Geometry: final body of the model. Coordinates: model frame, mm. Give positions to 0.01 mm unless a question says otherwise; leave off trailing zeros. One line per question, with ' | ' between items.
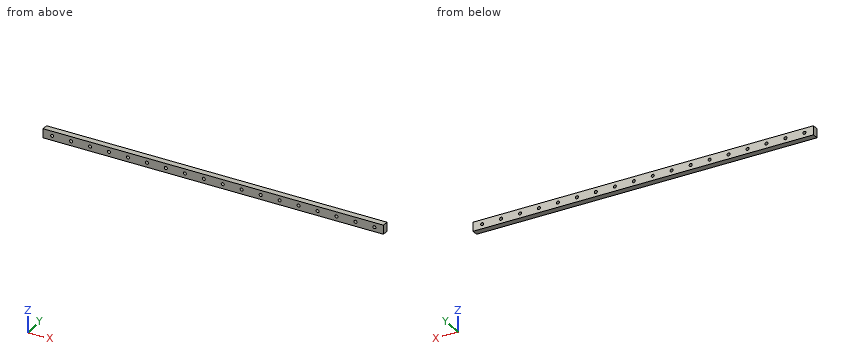
from build123d import *

# Parameters (mm, degrees)
SKETCH1_W           = 449
SKETCH1_H           = 12
SKETCH1_R           = 2
BOSS_EXTRUDE1_DEPTH = 8


with BuildPart() as part:
    # Sketch1 → Boss-Extrude1 (new body)
    with BuildSketch(Plane(origin=(0, 0, 0), x_dir=(1, 0, 0), z_dir=(0, 1, 0))):
        with Locations((224.5, 6)):
            Rectangle(SKETCH1_W, SKETCH1_H)
        with Locations(Location((12, 6, 0), (0, 0, 270))):
            Circle(SKETCH1_R, mode=Mode.SUBTRACT)
        with Locations(Location((37, 6, 0), (0, 0, 270))):
            Circle(SKETCH1_R, mode=Mode.SUBTRACT)
        with Locations(Location((62, 6, 0), (0, 0, 270))):
            Circle(SKETCH1_R, mode=Mode.SUBTRACT)
        with Locations(Location((87, 6, 0), (0, 0, 270))):
            Circle(SKETCH1_R, mode=Mode.SUBTRACT)
        with Locations(Location((112, 6, 0), (0, 0, 270))):
            Circle(SKETCH1_R, mode=Mode.SUBTRACT)
        with Locations(Location((137, 6, 0), (0, 0, 270))):
            Circle(SKETCH1_R, mode=Mode.SUBTRACT)
        with Locations(Location((162, 6, 0), (0, 0, 270))):
            Circle(SKETCH1_R, mode=Mode.SUBTRACT)
        with Locations(Location((187, 6, 0), (0, 0, 270))):
            Circle(SKETCH1_R, mode=Mode.SUBTRACT)
        with Locations(Location((212, 6, 0), (0, 0, 270))):
            Circle(SKETCH1_R, mode=Mode.SUBTRACT)
        with Locations(Location((237, 6, 0), (0, 0, 270))):
            Circle(SKETCH1_R, mode=Mode.SUBTRACT)
        with Locations(Location((262, 6, 0), (0, 0, 270))):
            Circle(SKETCH1_R, mode=Mode.SUBTRACT)
        with Locations(Location((287, 6, 0), (0, 0, 270))):
            Circle(SKETCH1_R, mode=Mode.SUBTRACT)
        with Locations(Location((312, 6, 0), (0, 0, 270))):
            Circle(SKETCH1_R, mode=Mode.SUBTRACT)
        with Locations(Location((337, 6, 0), (0, 0, 270))):
            Circle(SKETCH1_R, mode=Mode.SUBTRACT)
        with Locations(Location((362, 6, 0), (0, 0, 270))):
            Circle(SKETCH1_R, mode=Mode.SUBTRACT)
        with Locations(Location((387, 6, 0), (0, 0, 270))):
            Circle(SKETCH1_R, mode=Mode.SUBTRACT)
        with Locations(Location((412, 6, 0), (0, 0, 270))):
            Circle(SKETCH1_R, mode=Mode.SUBTRACT)
        with Locations(Location((437, 6, 0), (0, 0, 270))):
            Circle(SKETCH1_R, mode=Mode.SUBTRACT)
    extrude(amount=BOSS_EXTRUDE1_DEPTH)


solid = part.part
1) Material intervals for probe 1 along Z at (x, y) = (162, 5.75), sorted ascending. Write a range as from..to.
Check result:
probe 1: z = -12..-8, -4..0
2) Contact query for flat-ended pins moving along their axis: pin 1 Ø3 at (x, z) = (437, -6) entering from +Y; pin 2 Ø1.5 at (x, y) = (111, 6.5) entering from +Z. Output: stop coordinate, or through.
Check result:
pin 1: passes through | pin 2: stops at z = 0
3) Section A-A on y = 6.75. Count the separate pieces of the cut face and the enclosed holes in it, plus the area to 3 significant figures.
Check result:
separate pieces: 1 | enclosed holes: 18 | area: 5,160 mm^2
